Read the model definition and answer for the solid it produces. Units are mm, in the model's axes. A direction names the side the tool comes from. Round coordinates to 2 decimals unless told otherwise and drop trailing zeros. Order: outer loops, then holes, each group sorted by start corner. A loop starts at its lowest first (then second) coordinate and runs counter-clockwise, first axis right, second up. Notation, with made-up numbers: (-1.75, -10.75) -> (53.25, -10.75) arc R20 cw to (53.25, -5.75) -> close; hole circle Ø8 at (61.5, 47). An arc over 180 degrees is marked (long way). Answer as a JSON object with one key per item and string values. Group by question number.
Item 1: Given P1, Ø7, axis at x = -43.3, y = -17.5, coming from the +Z side (3 decimals); P2, Ø3, axis at y = 26, z = 7.5, coming from the +X side (3 decimals); P3, Ø1, axis at x = -50, y = -72, coming from the -Z side; P4, Ø5, axis at y = -8.5, z = 1.5, coming from the -X side (3 decimals), each flat-ended and moving along its own axis, determine where each tip first touches the part or whether it passes through.
Item 2: Section C-C, the plane y = -70 is taken. Write down the section's boundary in (x, z) (3 decimals), plus the area to 3 significant figures.
Item 3: For faces 1 (the cylindrical face through (-116.023, 67.161, -8.39)), 2 (the flat face through (-117, -1, -6.825)), 3 (the flat face through (117, -1, -6.825)), 4 (the flat face through (107.5, -1, 0)), 5 (the flat face through (115, -1, -10)), determine the directions among +Z, -Z, +X, -X, +Y, -Y from which every point of the face is accessible in a straight line to the end or side of a thin tool.
Item 4: Section D-D, the plane y = 61 is taken. Write down the section's boundary in (x, z) (3 decimals), plus the area to 3 significant figures.
Item 5: Consider probe 1 along Y at (x, z) = (-117.5, -8.7); probe 2 along X at (y, z) = (-62, 8.75) (3 decimals); probe 3 along Y at (x, z) = (92.3, 10.6). Determine where each line is inside the solid, lowest interval first. Write a range as from..to.
Item 6: The mould has two halves that part along X. Classify faces 6 (the flat face through (-110.675, -1, 3)), 7 (the cylindrical face through (118.977, 67.161, -8.39)), 8 (the flat face through (110.675, -1, 3)): pulls with the +X half, pulls with the -X half, needs draft (parallel to the pull), parting line crosses it, or undercut.
Item 7: Section B-B, the plane z = 5.25 is taken. Write down the section's boundary in (x, y) (3 decimals), plus the area to 3 significant figures.
Item 8: Section A-A, the plane x = -117.5 is taken. Write down the section's boundary in (y, z) (3 decimals), plus the area to 3 significant figures.
from build123d import *

# Parameters (mm, degrees)
F1_DEPTH      = 100
F2_R          = 3.2
F2_R_2        = 2.2
F3_DEPTH      = 10.001
F3_DEPTH_BACK = 13.176


with BuildPart() as f1:
    # F0 (on Front) → F1 (new body, symmetric)
    with BuildSketch(Plane.XZ):
        Polygon((-107.5, 10), (107.5, 10), (107.5, -10), (122.5, -10), (122.5, -6.825), (110.675, -6.825), (110.675, 13.175), (-110.675, 13.175), (-110.675, -6.825), (-122.5, -6.825), (-122.5, -10), (-107.5, -10), align=None)
    extrude(amount=F1_DEPTH, both=True)

    # F2 (on Top) → F3 (cut, two sides)
    with BuildSketch(Plane.XY) as f3_sk:
        with Locations((-117.5, -70)):
            Circle(F2_R)
        with Locations((-92.3, -17.5)):
            Circle(F2_R_2)
        with Locations((-55.3, -17.5)):
            Circle(F2_R_2)
        with Locations((-43.3, -17.5)):
            Circle(F2_R_2)
        with Locations((-6.3, -17.5)):
            Circle(F2_R_2)
        with Locations((6.3, -17.5)):
            Circle(F2_R_2)
        with Locations((43.3, -17.5)):
            Circle(F2_R_2)
        with Locations((55.3, -17.5)):
            Circle(F2_R_2)
        with Locations((92.3, -17.5)):
            Circle(F2_R_2)
        with Locations((117.5, -70)):
            Circle(F2_R)
        with Locations((-92.3, 17.5)):
            Circle(F2_R_2)
        with Locations((43.3, 17.5)):
            Circle(F2_R_2)
        with Locations((55.3, 17.5)):
            Circle(F2_R_2)
        with Locations((6.3, 17.5)):
            Circle(F2_R_2)
        with Locations((-6.3, 17.5)):
            Circle(F2_R_2)
        with Locations((-43.3, 17.5)):
            Circle(F2_R_2)
        with Locations((92.3, 17.5)):
            Circle(F2_R_2)
        with Locations((-55.3, 17.5)):
            Circle(F2_R_2)
        with Locations((-117.5, 70)):
            Circle(F2_R)
        with Locations((117.5, 70)):
            Circle(F2_R)
    extrude(amount=-F3_DEPTH, mode=Mode.SUBTRACT)
    extrude(f3_sk.sketch, amount=F3_DEPTH_BACK, mode=Mode.SUBTRACT)


solid = f1.part
Values found:
{
 "1": {"P1": "z = 13.175", "P2": "x = 110.675", "P3": "z = 10", "P4": "x = -110.675"},
 "2": {"outline": "(-122.5, -10) -> (-120.7, -10) -> (-120.7, -6.825) -> (-122.5, -6.825) -> close; (-114.3, -10) -> (-107.5, -10) -> (-107.5, 10) -> (107.5, 10) -> (107.5, -10) -> (114.3, -10) -> (114.3, -6.825) -> (110.675, -6.825) -> (110.675, 13.175) -> (-110.675, 13.175) -> (-110.675, -6.825) -> (-114.3, -6.825) -> close; (120.7, -10) -> (122.5, -10) -> (122.5, -6.825) -> (120.7, -6.825) -> close", "area": "864 mm2"},
 "3": {"face 1": "+Z, -Z", "face 2": "+Z, -X, +Y, -Y", "face 3": "+Z, +X, +Y, -Y", "face 4": "-Z, +Y, -Y", "face 5": "-Z, +X, -X, +Y, -Y"},
 "4": {"outline": "(-122.5, -10) -> (-107.5, -10) -> (-107.5, 10) -> (107.5, 10) -> (107.5, -10) -> (122.5, -10) -> (122.5, -6.825) -> (110.675, -6.825) -> (110.675, 13.175) -> (-110.675, 13.175) -> (-110.675, -6.825) -> (-122.5, -6.825) -> close", "area": "905 mm2"},
 "5": {"probe 1": "-100..-73.2, -66.8..66.8, 73.2..100", "probe 2": "-110.675..-107.5, 107.5..110.675", "probe 3": "-100..-19.7, -15.3..15.3, 19.7..100"},
 "6": {"face 6": "pulls with the -X half", "face 7": "undercut", "face 8": "pulls with the +X half"},
 "7": {"outline": "(-110.675, -100) -> (-107.5, -100) -> (-107.5, 100) -> (-110.675, 100) -> close; (107.5, -100) -> (110.675, -100) -> (110.675, 100) -> (107.5, 100) -> close", "area": "1,270 mm2"},
 "8": {"outline": "(-100, -10) -> (-73.2, -10) -> (-73.2, -6.825) -> (-100, -6.825) -> close; (-66.8, -10) -> (66.8, -10) -> (66.8, -6.825) -> (-66.8, -6.825) -> close; (73.2, -10) -> (100, -10) -> (100, -6.825) -> (73.2, -6.825) -> close", "area": "594 mm2"}
}
